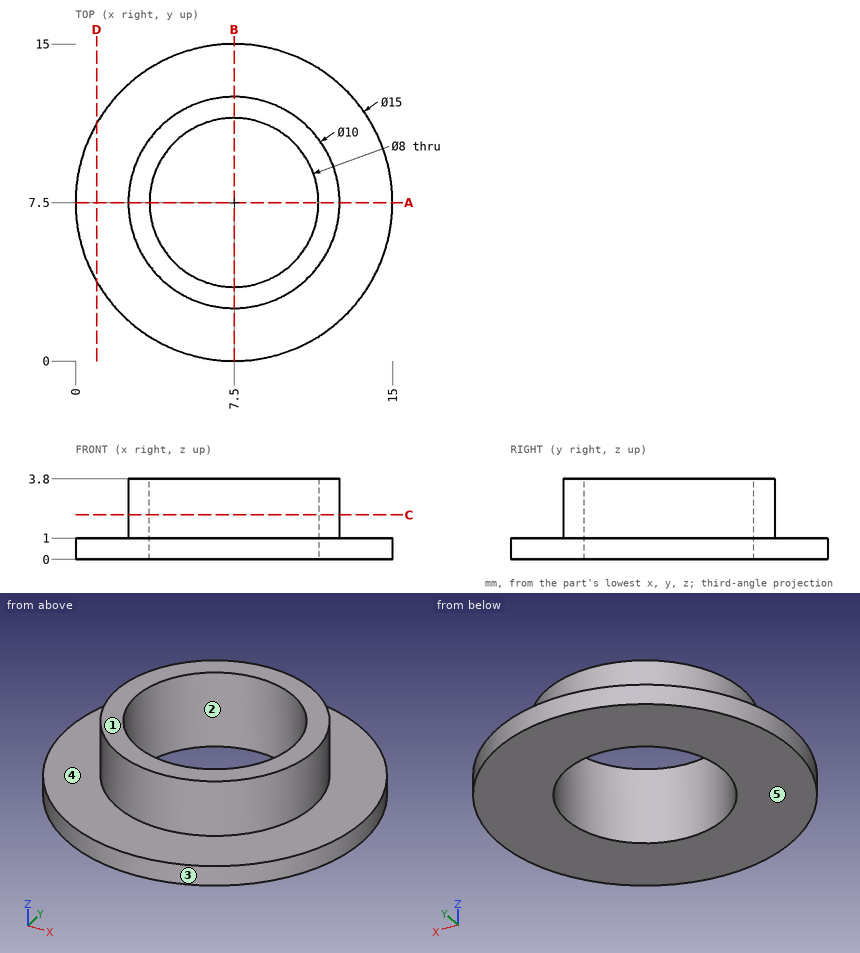
Geometry: see drawing. Coordinates: mm, zero at the bounding-box minimum. A direction names the side the tool comes from. Coordinates: 2 decimals unless noted, no trailing zeros. Loops run counter-clockwise (first coordinate to the right, second up) from the corner with the lowest first, then second, coordinate; pieces in that order, holes last. Notation, with made-up numbers: M 60,-7.75 L 78,-7.75 A12 ccw 78,15.25 Z; hole C 28.25,52 d6. An arc over 180 degrees is marked long. Answer in a Markdown table with one row per item.
1. Reachability of the marked faces 4 and 5 from +Z, -Z, +X, -X, +Y, -Y: full face, straight path, thin tool, end or side. Return the list, or none.
Response:
| item | result |
|---|---|
| face 4 | +Z |
| face 5 | -Z, +X, -X, +Y, -Y |
2. Section D-D, the plane x = 1. Output: boundary loops of the cut face in (y, z), then the cut area to 3 significant figures.
Response:
| item | result |
|---|---|
| outline | M 3.76,0 L 11.24,0 L 11.24,1 L 3.76,1 Z |
| area | 7.48 mm2 |
3. Section A-A, the plane y = 7.5. Output: boundary loops of the cut face in (x, z).
Response:
| item | result |
|---|---|
| outline | M 0,0 L 3.5,0 L 3.5,3.8 L 2.5,3.8 L 2.5,1 L 0,1 Z; M 11.5,0 L 15,0 L 15,1 L 12.5,1 L 12.5,3.8 L 11.5,3.8 Z |
4. Section C-C, the plane z = 2.1. Output: boundary loops of the cut face in (x, y).
Response:
| item | result |
|---|---|
| outline | C 7.5,7.5 d10; hole C 7.5,7.5 d8 |
5. Material intervals for line 1 (Y direction, x = 7.5, z = 2.9); line 2 (Z direction, x = 12.75, y = 3.5); line 3 (Y direction, x = 4, z = 0.6), sorted ascending.
Response:
| item | result |
|---|---|
| line 1 | y = 2.5 to 3.5, 11.5 to 12.5 |
| line 2 | z = 0 to 1 |
| line 3 | y = 0.87 to 5.56, 9.44 to 14.13 |
6. Draft query along Y for the marked faces 1, 2 and 3. Return one class per face: pulls with the +Y half, pulls with the -Y half, needs draft (parallel to the pull), parting line crosses it, or undercut.
Response:
| item | result |
|---|---|
| face 1 | needs draft |
| face 2 | undercut |
| face 3 | parting line crosses it |
7. First-contact query: pin 1 (1.5 mm diameter, centred on y = 3, z = 1, fed in from +X); pin 2 (2 mm diameter, centred on x = 2.5, z = 0.5, fed in from -Y); pin 3 (2 mm diameter, centred on x = 12, z = 2.5, fed in from -Y). Flat tips, straight axial feed; report the tip coordinate or a pass-through.
Response:
| item | result |
|---|---|
| pin 1 | stops at x = 14 |
| pin 2 | stops at y = 1.16 |
| pin 3 | stops at y = 3.93 |
